Check sheet for the modelled part. Datum: model origin and axes. Units: mm. Face numbers are marked on the shaded views. A direction names the side the tool comes from. Coordinates: 2 decimals unless noted, no trailing zeros. Order: outer loops, then holes, each group sorted by start corner. A loop starts at its lowest first (then second) coordinate and runs counter-clockwise, first axis right, second up.
from build123d import *

# Parameters (mm, degrees)
BASPROSKE_W        = 3
BASPROSKE_H        = 12.75
TOOTHCUT_DEPTH     = 19.27908641
TEETHCUTS_COUNT    = 15
TEETHCUTS_ANGLE    = 336
BORSKE_R           = 2.5
BORE_DEPTH         = 50.0000508
BOSS_EXTRU_1_DEPTH = 3


with BuildPart() as part:
    # BasProSke → Base-Revolve (revolve)
    with BuildSketch(Plane(origin=(0, 0, 0), x_dir=(1, 0, 0), z_dir=(0, 1, 0)), mode=Mode.PRIVATE) as base_revolve_sk:
        with Locations((1.5, 6.375)):
            Rectangle(BASPROSKE_W, BASPROSKE_H)
    revolve(base_revolve_sk.sketch.rotate(Axis((-10, 0, 0), (1, 0, 0)), 180), axis=Axis((-10, 0, 0), (1, 0, 0)))

    # TooCutSke → ToothCut (cut, through all)
    with BuildSketch(Plane(origin=(0, 0, 0), x_dir=(0, 0, -1), z_dir=(1, 0, 0))):
        with BuildLine():
            ThreePointArc((0.791546546, 9.340520867), (0, 9.374), (-0.791546546, 9.340520867))
            ThreePointArc((-0.791546546, 9.340520867), (-1.235070734, 11.110218102), (-2.344732916, 12.558386549))
            ThreePointArc((-2.344732916, 12.558386549), (0, 12.7754), (2.344732916, 12.558386549))
            ThreePointArc((2.344732916, 12.558386549), (1.235070734, 11.110218102), (0.791546546, 9.340520867))
        make_face()
    toothcut = extrude(amount=TOOTHCUT_DEPTH, mode=Mode.SUBTRACT)

    # TeethCuts: ToothCut ×15 about axis
    teethcuts_axis = Axis((-10, 0, 0), (1, 0, 0))
    for i in range(1, TEETHCUTS_COUNT):
        add(toothcut.rotate(teethcuts_axis, i * TEETHCUTS_ANGLE / (TEETHCUTS_COUNT - 1)), mode=Mode.SUBTRACT)

    # BorSke → Bore (cut, symmetric)
    with BuildSketch(Plane(origin=(0, 0, 0), x_dir=(0, 0, -1), z_dir=(1, 0, 0))):
        with Locations(Location((0, 0, 0), (0, 0, 180))):
            Circle(BORSKE_R)
    extrude(amount=BORE_DEPTH, both=True, mode=Mode.SUBTRACT)

    # Esquisse1 → Boss.-Extru.1 (add)
    with BuildSketch(Plane(origin=(3, 0, 0), x_dir=(0, 0, -1), z_dir=(1, 0, 0))):
        with BuildLine():
            Line((-2, 1.5), (-2, -1.5))
            ThreePointArc((-2, -1.5), (-2.5, 0), (-2, 1.5))
        make_face()
        with BuildLine():
            Line((2, 1.5), (2, -1.5))
            ThreePointArc((2, -1.5), (2.5, 0), (2, 1.5))
        make_face()
    extrude(amount=-BOSS_EXTRU_1_DEPTH)


solid = part.part
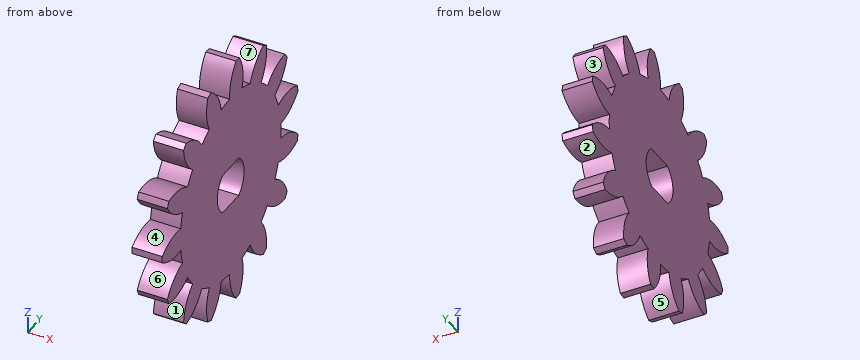
(1) Release check for a two-part mould opening along Y. For the marked faces 1, 2 and 3 record: +Y half, -Y half, draft (parallel to the pull), parting line (faces both ways), or undercut.
Filled in:
face 1: -Y half
face 2: undercut
face 3: +Y half
(2) Tool access check on the marked faces 4, 5, 6 and 7. Record the directions out of +Z, -Z, +X, -X, +Y, -Y that give a thin tool (end or side, any length) a straight path to the whole face; none if there is none.
Filled in:
face 4: +X, -X
face 5: -Z, +X, -X
face 6: +X, -X, -Y
face 7: +Z, +X, -X
(3) Go/stop test with flat-tipped pins: P1, Ø1.5, axis at x = 0.5, z = 7, coming from the +Y side; P2, Ø1.5, axis at x = 1, z = -6, coming from the -Y side. Record where each tip stops, or that it passes through.
Filled in:
P1: stops at y = 10.51
P2: stops at y = -11.62
(4) Cross-section at B-B (z = 10.25). Enter the section's corners in (x, y).
Filled in:
outline: (0, -4.49) - (3, -4.49) - (3, -2.05) - (0, -2.05) - close; (0, -0.16) - (3, -0.16) - (3, 2.3) - (0, 2.3) - close; (0, 4.67) - (3, 4.67) - (3, 6.69) - (0, 6.69) - close
(5) Cross-section at A-A (y = -10.75). Enter the section's corners in (x, z), and give its area (3 significant figures).
Filled in:
outline: (0, -5.6) - (3, -5.6) - (3, -3.63) - (0, -3.63) - close; (0, -1.18) - (3, -1.18) - (3, 1.18) - (0, 1.18) - close; (0, 3.63) - (3, 3.63) - (3, 5.6) - (0, 5.6) - close
area: 18.9 mm2
(6) Cross-section at C-C (y = -6). Enter the section's corners in (x, z), and give its area (3 significant figures).
Filled in:
outline: (0, -8.49) - (3, -8.49) - (3, 8.49) - (0, 8.49) - close
area: 50.9 mm2
(7) Thickness scan on probe 1 along Y at (x, z) = (1.25, 10.25); probe 2 along Z at (x, y) = (0.55, -8); probe 3 along Z at (x, y) = (2, 9.75). Record the ranges inside material, lowest first.
Filled in:
probe 1: y = -4.49 to -2.05, -0.16 to 2.3, 4.67 to 6.69
probe 2: z = -9.63 to -7.1, -4.89 to 4.89, 7.1 to 9.63
probe 3: z = -7.75 to -5.77, -3.33 to -0.83, 0.83 to 3.33, 5.77 to 7.75
